```python
from build123d import *

# Parameters (mm, degrees)
BOSS_EXTRUDE1_DEPTH             = 65
SKETCH2_R                       = 7.5
BOSS_EXTRUDE2_DEPTH             = 2.5
BOSS_EXTRUDE3_REACH             = 88.168
SKETCH3_W                       = 65
SKETCH3_H                       = 3
BOSS_EXTRUDE3_DIRECTION_2_REACH = 88.168
CUT_EXTRUDE2_REACH              = 124.042
SKETCH6_R                       = 1.75
CUT_EXTRUDE3_REACH              = 86.299
CUT_EXTRUDE4_REACH              = 86.299
FILLET1_R                       = 2.5
FILLET2_R                       = 5
CUT_EXTRUDE5_DEPTH              = 111.566722046
CUT_EXTRUDE5_DEPTH_BACK         = 111.566722046
SKETCH9_W                       = 12
SKETCH9_H                       = 32.949220019
SKETCH9_H_2                     = 17.949220019
BOSS_EXTRUDE5_DEPTH             = 22.8
SKETCH11_W                      = 18.75
SKETCH11_H                      = 16.8
CUT_EXTRUDE6_DEPTH              = 61.48
CHAMFER1_SIZE                   = 2.5
FILLET3_R                       = 5
FILLET4_R                       = 2.5
CUT_EXTRUDE8_REACH              = 112.567
SKETCH14_W                      = 3
SKETCH14_H                      = 5.1
CIRPATTERN1_START               = -40
CIRPATTERN1_OUTLINE_W           = 5.1
CIRPATTERN1_OUTLINE_H           = 3
CIRPATTERN1_DEPTH               = 25.3
CIRPATTERN1_START_2             = -2.55
CIRPATTERN1_2_OUTLINE_W         = 2.5
CIRPATTERN1_2_OUTLINE_H         = 3
CIRPATTERN1_2_DEPTH             = 5.1
CIRPATTERN1_START_3             = 37.5
CIRPATTERN1_3_OUTLINE_W         = 5.1
CIRPATTERN1_3_OUTLINE_H         = 3
CIRPATTERN1_3_DEPTH             = 2.5
CUT_EXTRUDE9_REACH              = 89.502
SKETCH15_W                      = 18.33254108
SKETCH15_H                      = 22.8


# Read off the part's stored shape, not the designer's step: CirPattern1
with BuildPart() as part:
    # Sketch1 → Boss-Extrude1 (new body)
    with BuildSketch(Plane.XY):
        Polygon((-40, 30), (-30, 40), (30, 40), (40, 30), (40, -30), (30, -40), (-30, -40), (-40, -30), align=None)
        Polygon((-37.5, 28.964466094), (-28.964466094, 37.5), (28.964466094, 37.5), (37.5, 28.964466094), (37.5, -28.964466094), (28.964466094, -37.5), (-28.964466094, -37.5), (-37.5, -28.964466094), align=None, mode=Mode.SUBTRACT)
    extrude(amount=BOSS_EXTRUDE1_DEPTH)

    # Sketch2 → Boss-Extrude2 (add)
    with BuildSketch(Plane.XY):
        Polygon((37.5, 28.964466094), (28.964466094, 37.5), (-28.964466094, 37.5), (-37.5, 28.964466094), (-37.5, -28.964466094), (-28.964466094, -37.5), (28.964466094, -37.5), (37.5, -28.964466094), align=None)
        Circle(SKETCH2_R, mode=Mode.SUBTRACT)
    extrude(amount=BOSS_EXTRUDE2_DEPTH)

    # Boss-Extrude3: up to this plane
    boss_extrude3_end = Plane(origin=(28.964466094, 37.5, 65), z_dir=(-0.7071067811865476, -0.7071067811865476, 0))
    # Sketch3 → Boss-Extrude3 (add, up to the surface)
    with BuildSketch(Plane(origin=(0, 0, 0), x_dir=(0, 0, -1), z_dir=(1, 0, 0)), mode=Mode.PRIVATE) as boss_extrude3_sk1:
        with Locations((-32.5, 31)):
            Rectangle(SKETCH3_W, SKETCH3_H)
    boss_extrude3_tool1 = split(extrude(boss_extrude3_sk1.sketch, amount=BOSS_EXTRUDE3_REACH, mode=Mode.PRIVATE), bisect_by=boss_extrude3_end, keep=Keep.BOTH, mode=Mode.PRIVATE)
    add(boss_extrude3_tool1.solids().sort_by_distance((0, 31, 32.5))[0])

    # Boss-Extrude3 direction 2: up to this plane
    boss_extrude3_direction_2_end = Plane(origin=(-37.5, 28.964466094, 65), z_dir=(0.707106781186547, -0.7071067811865481, 0))
    # Sketch3 → Boss-Extrude3 direction 2 (add, up to the surface)
    with BuildSketch(Plane(origin=(0, 0, 0), x_dir=(0, 0, -1), z_dir=(1, 0, 0)), mode=Mode.PRIVATE) as boss_extrude3_direction_2_sk1:
        with Locations((-32.5, 31)):
            Rectangle(SKETCH3_W, SKETCH3_H)
    boss_extrude3_direction_2_tool1 = split(extrude(boss_extrude3_direction_2_sk1.sketch, amount=-BOSS_EXTRUDE3_DIRECTION_2_REACH, mode=Mode.PRIVATE), bisect_by=boss_extrude3_direction_2_end, keep=Keep.BOTH, mode=Mode.PRIVATE)
    add(boss_extrude3_direction_2_tool1.solids().sort_by_distance((0, 31, 32.5))[0])

    # Sketch6 → Cut-Extrude2 (cut, up to next)
    with BuildSketch(Plane(origin=(0, 29.5, -27), x_dir=(-1, 0, 0), z_dir=(0, -1, 0)), mode=Mode.PRIVATE) as cut_extrude2_sk1:
        with Locations(Location((-4.5, -72, 0), (0, 0, 90))):
            Circle(SKETCH6_R)
    cut_extrude2_tool1 = extrude(cut_extrude2_sk1.sketch, amount=-CUT_EXTRUDE2_REACH, mode=Mode.PRIVATE) & part.part
    # Sketch6 → Cut-Extrude2 (cut, up to next)
    with BuildSketch(Plane(origin=(0, 29.5, -27), x_dir=(-1, 0, 0), z_dir=(0, -1, 0)), mode=Mode.PRIVATE) as cut_extrude2_sk2:
        with Locations(Location((25.5, -37, 0), (0, 0, 90))):
            Circle(SKETCH6_R)
    cut_extrude2_tool2 = extrude(cut_extrude2_sk2.sketch, amount=-CUT_EXTRUDE2_REACH, mode=Mode.PRIVATE) & part.part
    add(cut_extrude2_tool1.solids().sort_by_distance((4.5, 29.5, 45))[0], mode=Mode.SUBTRACT)
    add(cut_extrude2_tool2.solids().sort_by_distance((-25.5, 29.5, 10))[0], mode=Mode.SUBTRACT)

    # Sketch7 → Cut-Extrude3 (cut, up to next)
    with BuildSketch(Plane.XY.offset(2.5), mode=Mode.PRIVATE) as cut_extrude3_sk1:
        Polygon((-33.964466094, 32.5), (-28.964466094, 37.5), (28.964466094, 37.5), (33.964466094, 32.5), align=None)
    cut_extrude3_tool1 = extrude(cut_extrude3_sk1.sketch, amount=-CUT_EXTRUDE3_REACH, mode=Mode.PRIVATE) & part.part
    add(cut_extrude3_tool1.solids().sort_by_distance((0, 34.933788, 2.5))[0], mode=Mode.SUBTRACT)

    # Sketch8 → Cut-Extrude4 (cut, up to next)
    with BuildSketch(Plane.XY.offset(2.5), mode=Mode.PRIVATE) as cut_extrude4_sk1:
        Polygon((-7.5, 0), (-7.5, 11), (-10.5, 11), (-20.5, 11), (-20.5, 20), (-0.5, 20), (-0.5, 7.5), (0, 7.5), align=None)
    cut_extrude4_tool1 = extrude(cut_extrude4_sk1.sketch, amount=-CUT_EXTRUDE4_REACH, mode=Mode.PRIVATE) & part.part
    add(cut_extrude4_tool1.solids().sort_by_distance((-9.150457, 13.572273, 2.5))[0], mode=Mode.SUBTRACT)

    # Fillet1
    fillet1_edges = [part.edges().sort_by_distance(p)[0] for p in [
        (-20.5, 11, 1.25),
        (-20.5, 20, 1.25),
        (-0.5, 20, 1.25),
    ]]
    fillet(fillet1_edges, radius=FILLET1_R)

    # Fillet2
    fillet2_edges = [part.edges().sort_by_distance(p)[0] for p in [
        (-0.5, 7.5, 1.25),
        (-7.5, 11, 1.25),
    ]]
    fillet(fillet2_edges, radius=FILLET2_R)

    # Sketch9 → Cut-Extrude5 (cut, two sides: drawn at the far end of the back side and taken through both)
    with BuildSketch(Plane(origin=(0, 40, 0), x_dir=(1, 0, 0), z_dir=(0, 1, 0)).offset(-CUT_EXTRUDE5_DEPTH_BACK)):
        with Locations((24, -66.474610009)):
            Rectangle(SKETCH9_W, SKETCH9_H)
        with Locations((-24, -58.97461001)):
            Rectangle(SKETCH9_W, SKETCH9_H_2)
    extrude(amount=CUT_EXTRUDE5_DEPTH + CUT_EXTRUDE5_DEPTH_BACK, mode=Mode.SUBTRACT)

    # Sketch10 → Boss-Extrude5 (add)
    with BuildSketch(Plane(origin=(0, -37.5, 0), x_dir=(1, 0, 0), z_dir=(0, 1, 0))):
        with BuildLine():
            Line((-4.70239318, -35.65016071), (-21.95239318, -35.65016071))
            ThreePointArc((-21.95239318, -35.65016071), (-23.013053352, -35.210820882), (-23.45239318, -34.15016071))
            Line((-23.45239318, -34.15016071), (-23.45239318, -27.14854667))
            ThreePointArc((-23.45239318, -27.14854667), (-23.013053352, -26.087886498), (-21.95239318, -25.64854667))
            Line((-21.95239318, -25.64854667), (20.04760682, -25.64854667))
            ThreePointArc((20.04760682, -25.64854667), (21.108266992, -26.087886498), (21.54760682, -27.14854667))
            Line((21.54760682, -27.14854667), (21.54760682, -34.15016071))
            ThreePointArc((21.54760682, -34.15016071), (21.108266992, -35.210820882), (20.04760682, -35.65016071))
            Line((20.04760682, -35.65016071), (2.79760682, -35.65016071))
            Line((2.79760682, -35.65016071), (2.79760682, -53.98270179))
            Line((2.79760682, -53.98270179), (10.59521364, -53.98270179))
            ThreePointArc((10.59521364, -53.98270179), (11.655873812, -54.422041618), (12.09521364, -55.48270179))
            Line((12.09521364, -55.48270179), (12.09521364, -62.48))
            ThreePointArc((12.09521364, -62.48), (11.655873812, -63.540660172), (10.59521364, -63.98))
            Line((10.59521364, -63.98), (-12.5, -63.98))
            ThreePointArc((-12.5, -63.98), (-13.560660172, -63.540660172), (-14, -62.48))
            Line((-14, -62.48), (-14, -55.48270179))
            ThreePointArc((-14, -55.48270179), (-13.560660172, -54.422041618), (-12.5, -53.98270179))
            Line((-12.5, -53.98270179), (-4.70239318, -53.98270179))
            Line((-4.70239318, -53.98270179), (-4.70239318, -35.65016071))
        make_face()
    extrude(amount=BOSS_EXTRUDE5_DEPTH)

    # Sketch11 → Cut-Extrude6 (cut)
    with BuildSketch(Plane.XY.offset(63.98)):
        with Locations((-14.07739318, -26.1)):
            Rectangle(SKETCH11_W, SKETCH11_H)
        with Locations((12.17260682, -26.1)):
            Rectangle(SKETCH11_W, SKETCH11_H)
    extrude(amount=-CUT_EXTRUDE6_DEPTH, mode=Mode.SUBTRACT)

    # Chamfer1
    chamfer1_edges = [part.edges().sort_by_distance(p)[0] for p in [
        (0, 40, 65),
        (0, -40, 65),
    ]]
    chamfer(chamfer1_edges, length=CHAMFER1_SIZE - 0.0001)  # a hair under: the kernel refuses the full size

    # Fillet3
    fillet3_edges = [part.edges().sort_by_distance(p)[0] for p in [
        (-4.70239318, -17.7, 30.64935369),
        (-4.70239318, -34.5, 30.64935369),
        (-4.70239318, -34.5, 58.981350895),
        (2.79760682, -34.5, 58.981350895),
        (2.79760682, -34.5, 30.64935369),
        (2.79760682, -17.7, 30.64935369),
    ]]
    fillet(fillet3_edges, radius=FILLET3_R)

    # Fillet4
    fillet4_edges = [part.edges().sort_by_distance(p)[0] for p in [
        (-4.70239318, -17.7, 58.981350895),
        (2.79760682, -17.7, 58.981350895),
    ]]
    fillet(fillet4_edges, radius=FILLET4_R)

    # Sketch14 → Cut-Extrude8 (cut, up to next)
    with BuildSketch(Plane(origin=(40, 0, 0), x_dir=(0, 0, -1), z_dir=(1, 0, 0)), mode=Mode.PRIVATE) as cut_extrude8_sk1:
        with Locations((-48.5, 0)):
            Rectangle(SKETCH14_W, SKETCH14_H)
    cut_extrude8_tool1 = extrude(cut_extrude8_sk1.sketch, amount=-CUT_EXTRUDE8_REACH, mode=Mode.PRIVATE) & part.part
    # Sketch14 → Cut-Extrude8 (cut, up to next)
    with BuildSketch(Plane(origin=(40, 0, 0), x_dir=(0, 0, -1), z_dir=(1, 0, 0)), mode=Mode.PRIVATE) as cut_extrude8_sk2:
        with Locations((-16.5, 0)):
            Rectangle(SKETCH14_W, SKETCH14_H)
    cut_extrude8_tool2 = extrude(cut_extrude8_sk2.sketch, amount=-CUT_EXTRUDE8_REACH, mode=Mode.PRIVATE) & part.part
    add(cut_extrude8_tool1.solids().sort_by_distance((40, 0, 48.5))[0], mode=Mode.SUBTRACT)
    add(cut_extrude8_tool2.solids().sort_by_distance((40, 0, 16.5))[0], mode=Mode.SUBTRACT)

    # CirPattern1 outline → CirPattern1 (cut)
    with BuildSketch(Plane(origin=(0, 0, 0), x_dir=(1, 0, 0), z_dir=(0, 1, 0)).offset(CIRPATTERN1_START)):
        with Locations((0, -16.5)):
            Rectangle(CIRPATTERN1_OUTLINE_W, CIRPATTERN1_OUTLINE_H)
        with Locations((0, -48.5)):
            Rectangle(CIRPATTERN1_OUTLINE_W, CIRPATTERN1_OUTLINE_H)
    extrude(amount=CIRPATTERN1_DEPTH, mode=Mode.SUBTRACT)

    # CirPattern1 2 outline → CirPattern1 2 (cut)
    with BuildSketch(Plane(origin=(0, 0, 0), x_dir=(1, 0, 0), z_dir=(0, 1, 0)).offset(CIRPATTERN1_START_2)):
        with Locations((-38.75, -16.5)):
            Rectangle(CIRPATTERN1_2_OUTLINE_W, CIRPATTERN1_2_OUTLINE_H)
        with Locations((-38.75, -48.5)):
            Rectangle(CIRPATTERN1_2_OUTLINE_W, CIRPATTERN1_2_OUTLINE_H)
    extrude(amount=CIRPATTERN1_2_DEPTH, mode=Mode.SUBTRACT)

    # CirPattern1 3 outline → CirPattern1 3 (cut)
    with BuildSketch(Plane(origin=(0, 0, 0), x_dir=(1, 0, 0), z_dir=(0, 1, 0)).offset(CIRPATTERN1_START_3)):
        with Locations((0, -16.5)):
            Rectangle(CIRPATTERN1_3_OUTLINE_W, CIRPATTERN1_3_OUTLINE_H)
        with Locations((0, -48.5)):
            Rectangle(CIRPATTERN1_3_OUTLINE_W, CIRPATTERN1_3_OUTLINE_H)
    extrude(amount=CIRPATTERN1_3_DEPTH, mode=Mode.SUBTRACT)

    # Sketch15 → Cut-Extrude9 (cut, up to next)
    with BuildSketch(Plane(origin=(2.79760682, 0, 0), x_dir=(0, 0, -1), z_dir=(1, 0, 0)), mode=Mode.PRIVATE) as cut_extrude9_sk1:
        with Locations((-44.81643125, -26.1)):
            Rectangle(SKETCH15_W, SKETCH15_H)
    cut_extrude9_tool1 = extrude(cut_extrude9_sk1.sketch, amount=-CUT_EXTRUDE9_REACH, mode=Mode.PRIVATE) & part.part
    add(cut_extrude9_tool1.solids().sort_by_distance((2.797607, -26.1, 44.816431))[0], mode=Mode.SUBTRACT)


solid = part.part
```
For this review, take the finished solid that the model builds, in its own axes (mm). A direction names the side the tool comes from. Round coordinates to 2 decimals unless told otherwise and drop trailing zeros. Loops run counter-clockwise (first coordinate to the right, second up) from the corner with the lowest first, then second, coordinate; pieces in that order, holes last.
Q1. Add section C-C on z = 10. Write out the cut boundary in (x, y), plus the area to 3 significant figures.
Result sheet:
outline: (-40, -30) - (-30, -40) - (30, -40) - (40, -30) - (40, 30) - (30, 40) - (-30, 40) - (-40, 30) - close; hole (-37.5, -28.96) - (-28.96, -37.5) - (28.96, -37.5) - (37.5, -28.96) - (37.5, 28.96) - (36.96, 29.5) - (-23.75, 29.5) - (-23.75, 32.5) - (33.96, 32.5) - (28.96, 37.5) - (-28.96, 37.5) - (-33.96, 32.5) - (-27.25, 32.5) - (-27.25, 29.5) - (-36.96, 29.5) - (-37.5, 28.96) - close
area: 923 mm2
Q2. To check wall thickness, follow line 1 along Y through (x, z) = (14.5, 52.5); line 2 along Y through (x, z) = (15, 26); line 3 along X through (y, z) = (-15, 33). State the ranges of each line that lie inside material, in increasing order.
Result sheet:
line 1: y = -40 to -37.5, 29.5 to 32.5, 37.5 to 40
line 2: y = -40 to -34.5, -17.7 to -14.7, 29.5 to 32.5, 37.5 to 40
line 3: x = -40 to -37.5, -23.45 to 21.55, 37.5 to 40
Q3. Machinability: for faces 4 (the face through (0, 39, 18)), 5 (the face through (-20.5, 15, 1)), 6 (the face through (-30, 31, 58)), 7 (the face through (4.223, -32.996, 30.579)), which of the approach directions +Z, -Z, +X, -X, +Y, -Y give a long, thin tool a straight path to every point of the face, cutting with its end or side? Answer none if there is none.
Result sheet:
face 4: +Y
face 5: +Z, -Z
face 6: +Z, +Y, -Y
face 7: +Z
Q4. Add section A-A on x = -25.5. Write out the cut boundary in (y, z), plus the area to 3 significant figures.
Result sheet:
outline: (-40, 0) - (32.5, 0) - (32.5, 8.25) - (29.5, 8.25) - (29.5, 2.5) - (-37.5, 2.5) - (-37.5, 50) - (-40, 50) - close; (29.5, 11.75) - (32.5, 11.75) - (32.5, 50) - (29.5, 50) - close; (37.5, 0) - (40, 0) - (40, 50) - (37.5, 50) - close
area: 557 mm2
Q5. Mouldability with a two-part tool opening along Z and no side actions: class faces 1 (the face through (-4.702, -25, 59)), 2 (the face through (-24, 31, 50)), 3 (the face through (-39, 2.55, 48)) as +Z half, -Z half, draft (parallel to the pull), parting line (faces both ways), or undercut.
Result sheet:
face 1: draft
face 2: +Z half
face 3: undercut
Q6. Add section D-D on y = -21.5. Write out the cut boundary in (x, z).
Result sheet:
outline: (-40, 0) - (40, 0) - (40, 65) - (37.5, 65) - (37.5, 2.5) - (-37.5, 2.5) - (-37.5, 65) - (-40, 65) - close; (-4.85, 25.65) - (2.94, 25.65) - (2.94, 35.65) - (-4.85, 35.65) - close; (-4.7, 53.98) - (2.8, 53.98) - (2.8, 63.98) - (-4.7, 63.98) - close
Q7. Add section B-B on x = 32.5. Write out the cut boundary in (y, z), plus the area to 3 significant figures.
Result sheet:
outline: (-37.5, 0) - (32.5, 0) - (32.5, 65) - (29.5, 65) - (29.5, 2.5) - (-33.96, 2.5) - (-33.96, 65) - (-37.5, 65) - close; (33.96, 0) - (37.5, 0) - (37.5, 65) - (33.96, 65) - close
area: 813 mm2
Q8. Insertion check: pin 1 Ø0.8 at (y, z) = (-39, 58) entering from -X; pin 2 Ø11.5 at (x, y) = (-4.5, -21.5) entering from +Z; pin 3 Ø3 at (y, z) = (38.5, 48) entering from -X. Each pin has a flat end and moves straight along its axis. Give the tip position at first contact, or say it passes through.
Result sheet:
pin 1: stops at x = -31.4
pin 2: stops at z = 63.98
pin 3: stops at x = -33
